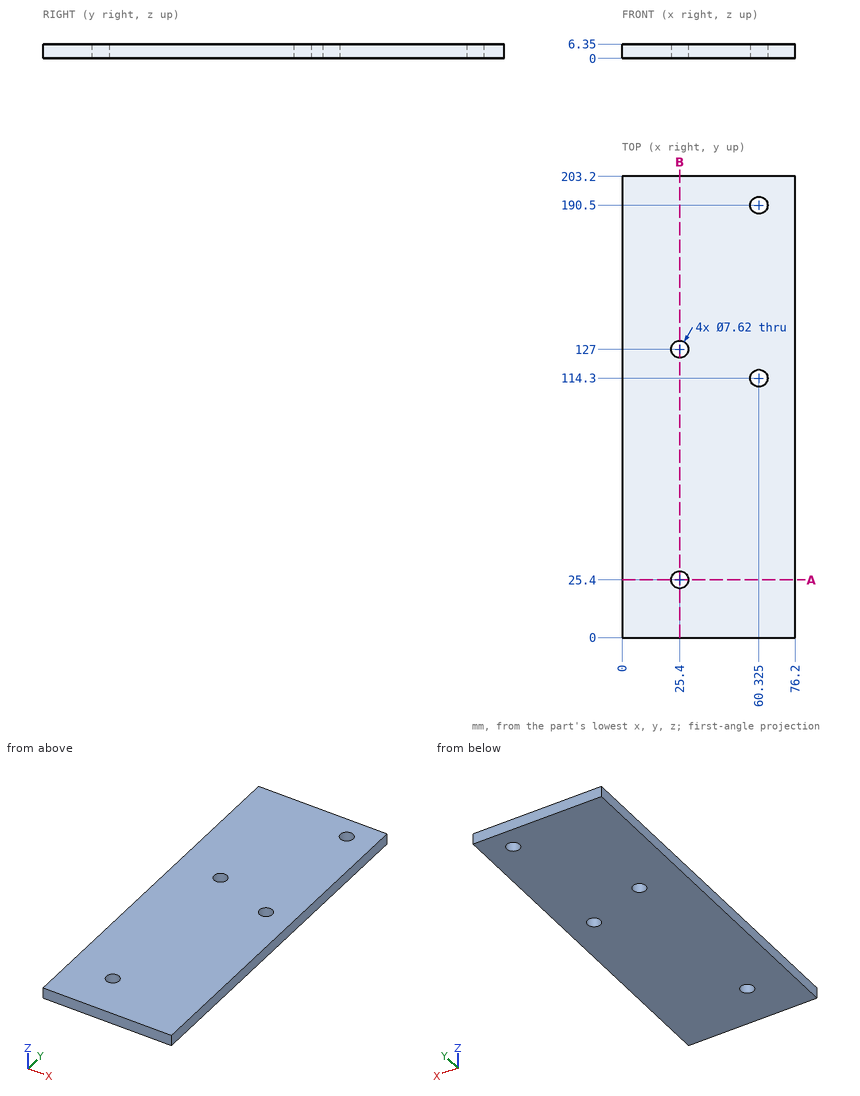
The figure shows three views and two pictorial views of one solid part (mm, origin at its lowest corner). Answer the questions. Round coordinates to 2 decimals unless told otherwise and drop trailing zeros. Write each loop counter-clockwise with the first axis right and the second up, starting at its lowest first coordinate (ties: lowest second). Pieces come first, ordered by that corner, then holes. Notation, with made-up numbers: (12, 79.25) -> (21, 79.25) arc R29 cw to (21, 107.25) -> close; hole circle Ø10 at (-4, 81.25). An arc over 180 degrees is marked (long way). Answer as a JSON object with one key per item and string values. Group by question number.
Q1. Section B-B (x = 25.4) is taken. Write down the section's boundary in (y, z), plus the area to 3 significant figures.
Q2. This flat-tipped pin is pushed along its axis until it touches: pin 1 Ø7 at (x, y) = (25.4, 25.4) entering from -Z. Where does it stop, or does it pass through?
Q3. Straight lines are drawn through the part: line 1 along Y through (x, z) = (25.4, 2); line 2 along X through (y, z) = (114.3, 3.5) (3 decimals); line 3 along X through (y, z) = (25.4, 4.5). For each, find the intervals that lie inside material, in ascending order.
Q4. Section A-A (y = 25.4) is taken. Write down the section's boundary in (x, z), plus the area to 3 significant figures.
Check values:
{
 "1": {"outline": "(0, 0) -> (21.59, 0) -> (21.59, 6.35) -> (0, 6.35) -> close; (29.21, 0) -> (123.19, 0) -> (123.19, 6.35) -> (29.21, 6.35) -> close; (130.81, 0) -> (203.2, 0) -> (203.2, 6.35) -> (130.81, 6.35) -> close", "area": "1,190 mm^2"},
 "2": {"pin 1": "through"},
 "3": {"line 1": "0 to 21.59, 29.21 to 123.19, 130.81 to 203.2", "line 2": "0 to 56.515, 64.135 to 76.2", "line 3": "0 to 21.59, 29.21 to 76.2"},
 "4": {"outline": "(0, 0) -> (21.59, 0) -> (21.59, 6.35) -> (0, 6.35) -> close; (29.21, 0) -> (76.2, 0) -> (76.2, 6.35) -> (29.21, 6.35) -> close", "area": "435 mm^2"}
}
